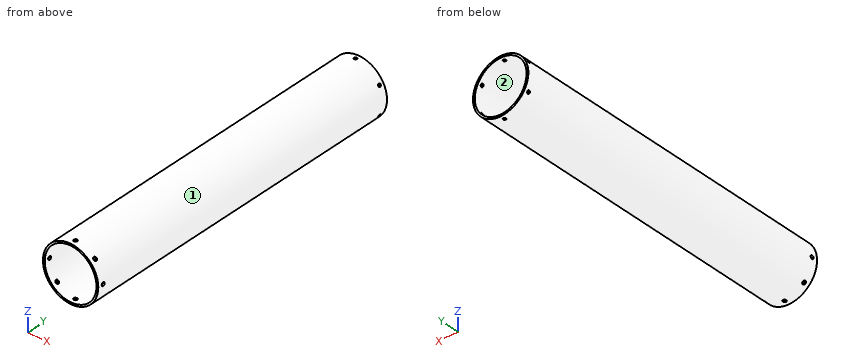
```python
from build123d import *

# Parameters (mm, degrees)
SKETCH2_R           = 19.25
SKETCH2_R_2         = 18
BOSS_EXTRUDE1_DEPTH = 231.82
SKETCH3_R           = 1.205
CUT_EXTRUDE2_DEPTH  = 231.82
CIRPATTERN3_COUNT   = 8
SKETCH4_R           = 0.991990711
CUT_EXTRUDE3_DEPTH  = 231.82
CIRPATTERN4_COUNT   = 6


with BuildPart() as part:
    # Sketch2 → Boss-Extrude1 (new body)
    with BuildSketch(Plane(origin=(0, 0, 0), x_dir=(1, 0, 0), z_dir=(0, 1, 0))):
        Circle(SKETCH2_R)
        Circle(SKETCH2_R_2, mode=Mode.SUBTRACT)
    extrude(amount=BOSS_EXTRUDE1_DEPTH)

    # Sketch3 → Cut-Extrude2 (cut)
    with BuildSketch(Plane.XY):
        with Locations((0, 3.92)):
            Circle(SKETCH3_R)
    cut_extrude2 = extrude(amount=-CUT_EXTRUDE2_DEPTH, mode=Mode.SUBTRACT)

    # CirPattern3: Cut-Extrude2 ×8 about axis
    cirpattern3_axis = Axis((0, 231.82, 0), (0, -1, 0))
    for i in range(1, CIRPATTERN3_COUNT):
        add(cut_extrude2.rotate(cirpattern3_axis, i * 360 / CIRPATTERN3_COUNT), mode=Mode.SUBTRACT)

    # Sketch4 → Cut-Extrude3 (cut)
    with BuildSketch(Plane.XY):
        with Locations((0, 228.73)):
            Circle(SKETCH4_R)
    cut_extrude3 = extrude(amount=CUT_EXTRUDE3_DEPTH, mode=Mode.SUBTRACT)

    # CirPattern4: Cut-Extrude3 ×6 about axis
    cirpattern4_axis = Axis((0, 231.82, 0), (0, -1, 0))
    for i in range(1, CIRPATTERN4_COUNT):
        add(cut_extrude3.rotate(cirpattern4_axis, i * 360 / CIRPATTERN4_COUNT), mode=Mode.SUBTRACT)


solid = part.part
```
Part model, mm, in its own coordinate system. Face numbers are marked on the shaded views. Round coordinates to 2 decimals unless told otherwise and drop trailing zeros. Order: outer loops, then holes, each group sorted by start corner. A loop starts at its lowest first (then second) coordinate and runs counter-clockwise, first axis right, second up. Notation, with made-up numbers: M -35,63 L 18,63 A21 cw 18,96 Z; hole C 65,36.5 d8. An arc over 180 degrees is marked long. Answer in a Markdown table with one row per item. Add a question column.
Q1. Cut at C-C on y = 147. Give the cut face in (x, z).
Q2. Pin check, flat tips, straight feed: pin 1 (1.5 mm diameter, centred on x = 2.5, y = 34.5, fed in from +Z); pin 2 (12 mm diameter, centred on x = -11, y = 125.5, fed in from +Z); pin 3 (8 mm diameter, centred on x = 5.5, y = 80.5, fed in from -Z). Stop position of each tip, or through.
Q3. Cut at A-A on x = 6.5. Give the cut face in (y, z).
Q4. Mould opens along X. For the marked faces 1 and 2 say: +X half, -X half, draft (parallel to the pull), parting line (faces both ways), or undercut.
Q5. Cut at B-B on z = -4.5. Give the cut face in (x, y), and give its area (3 significant figures).
Q6. Wall check: L1, parallel to Y at x = 0, z = 18.3 (3 decimals); L2, parallel to Z at x = -1, y = 57.5; L3, parallel to Y at x = 13, z = 13 (3 decimals). Give the ranges that are in metal, low to high. Write a range as from..to.
Established:
| question | item | result |
|---|---|---|
| 1 | outline | C 0,0 d38.5; hole C 0,0 d36 |
| 2 | pin 1 | stops at z = 19.17 |
| 2 | pin 2 | stops at z = 18.59 |
| 2 | pin 3 | stops at z = -19.19 |
| 3 | outline | M 0,-18.12 L 231.82,-18.12 L 231.82,-16.79 L 0,-16.79 Z; M 0,16.79 L 231.82,16.79 L 231.82,18.12 L 0,18.12 Z |
| 4 | face 1 | parting line |
| 4 | face 2 | undercut |
| 5 | outline | M -18.72,0 L -17.43,0 L -17.43,231.82 L -18.72,231.82 Z; M 17.43,0 L 18.72,0 L 18.72,231.82 L 17.43,231.82 Z |
| 5 | area | 597 mm2 |
| 6 | L1 | y = 0..2.715, 5.125..227.738, 229.722..231.82 |
| 6 | L2 | z = -19.22..-17.97, 17.97..19.22 |
| 6 | L3 | y = 0..2.715, 5.125..231.82 |
